```python
from build123d import *

# Parameters (mm, degrees)
F0_W     = 51
F0_H     = 30
F1_DEPTH = 3.175
F2_W     = 115.3
F2_H     = 72.9
F4_DEPTH = 25.4
F3_W     = 115.3
F3_H     = 72.9
F5_DEPTH = 25.4
F6_R     = 0.5
F7_DEPTH = 25


with BuildPart() as f1:
    # F0 (on Top) → F1 (new body)
    with BuildSketch(Plane.XY):
        with BuildLine():
            Line((61, 42.8), (-61, 42.8))
            ThreePointArc((-61, 42.8), (-63.1213203436, 41.9213203436), (-64, 39.8))
            Line((-64, 39.8), (-64, -39.8))
            ThreePointArc((-64, -39.8), (-63.1213203436, -41.9213203436), (-61, -42.8))
            Line((-61, -42.8), (61, -42.8))
            ThreePointArc((61, -42.8), (63.1213203436, -41.9213203436), (64, -39.8))
            Line((64, -39.8), (64, 39.8))
            ThreePointArc((64, 39.8), (63.1213203436, 41.9213203436), (61, 42.8))
        make_face()
        Rectangle(F0_W, F0_H, mode=Mode.SUBTRACT)
    extrude(amount=F1_DEPTH)

    # F2 (on Top) → F4 (join)
    with BuildSketch(Plane.XY):
        with BuildLine():
            Line((-63.9396576047, -36.1556038049), (-57.5896576047, -36.1556038049))
            Line((-57.5896576047, -36.1556038049), (-57.5896576047, -42.5056038049))
            Line((-57.5896576047, -42.5056038049), (61.0603423953, -42.5056038049))
            ThreePointArc((61.0603423953, -42.5056038049), (63.1816627389, -41.6269241484), (64.0603423953, -39.5056038049))
            Line((64.0603423953, -39.5056038049), (64.0603423953, -36.1556038049))
            Line((64.0603423953, -36.1556038049), (64.0603423953, 36.7443961951))
            Line((64.0603423953, 36.7443961951), (64.0603423953, 40.0943961951))
            ThreePointArc((64.0603423953, 40.0943961951), (63.1816627389, 42.2157165387), (61.0603423953, 43.0943961951))
            Line((61.0603423953, 43.0943961951), (-57.5896576047, 43.0943961951))
            Line((-57.5896576047, 43.0943961951), (-60.9396576047, 43.0943961951))
            ThreePointArc((-60.9396576047, 43.0943961951), (-63.0609779483, 42.2157165387), (-63.9396576047, 40.0943961951))
            Line((-63.9396576047, 40.0943961951), (-63.9396576047, -36.1556038049))
        make_face()
        with Locations((0.0603423953, 0.2943961951)):
            Rectangle(F2_W, F2_H, mode=Mode.SUBTRACT)
        with Locations((0.0603423953, 0.2943961951)):
            Rectangle(F2_W, F2_H)
    extrude(amount=-F4_DEPTH)

    # F3 (on Top) → F5 (cut)
    with BuildSketch(Plane.XY):
        Rectangle(F3_W, F3_H)
    extrude(amount=-F5_DEPTH, mode=Mode.SUBTRACT)

    # F6 (on face) → F7 (cut)
    with BuildSketch(Plane(origin=(0, 43.0943961951, 0), x_dir=(-1, 0, 0), z_dir=(0, 1, 0))):
        with Locations((0, -14.8937767372)):
            Circle(F6_R)
    extrude(amount=-F7_DEPTH, mode=Mode.SUBTRACT)


solid = f1.part
```
Geometry check sheet. Reference: the model listing, model coordinates, mm. A direction names the side the tool comes from. Coordinates: 2 decimals unless noted, no trailing zeros. Write each loop counter-clockwise with the first axis right and the second up, starting at its lowest first coordinate (ties: lowest second). Pieces come first, ordered by that corner, then holes. Notation, with made-up numbers: M 51,-18.75 L 109,-18.75 A17 cw 109,12.25 Z; hole C -11.75,-30.5 d2. An arc over 180 degrees is marked long. Use one line per item in the form item = value. Start each with the question number.
1) Section check D-D on z = -3. Enter the section's corners in (x, y).
2) Thickness scan on probe 1 along X at (y, z) = (-15.5, -4.5); probe 2 along Y at (x, z) = (-28, -21.75); probe 3 along Z at (x, y) = (0, 41.75) (3 decimals). Record the ranges inside material, lowest first. Write a range as from..to.
3) Section check C-C on y = 35. Enter the section's corners in (x, z) (3 decimals), and give its area (3 significant figures).
4) Go/stop test with flat-tipped pins: pin 1 Ø7.5 at (x, z) = (-27, -9.5) entering from -Y; pin 2 Ø1 at (y, z) = (-9.5, 1) entering from +X; pin 3 Ø6 at (x, y) = (40.5, -33) entering from -Z. Record where each tip stops, or that it passes through.
5) Section check B-B on x = -44.5. Enter the section's corners in (y, z) (3 decimals), and give its area (3 significant figures).
6) Section check A-A on x = -13.5. Enter the section's corners in (y, z) (3 decimals).
7) Set-up check for faces 5 (the flat face through (1, -42.506, -13)), 6 (the cylindrical face through (63.14, 41.9, 1.57)), 7 (the flat face through (25.5, 0, 2)), 8 (the flat face through (-57.59, -39, -13)), 9 (the cylindrical face through (-63.1, 41.94, 1.57)): record each of +Z, -Z, +X, -X, +Y, -Y from which the full face is reachable in a straight line by a thin tool's end or side.
8) Release check for a two-part mould opening along X. For faces 1 (the flat face through (-57.65, 0, -13)), 2 (the cylindrical face through (-63.14, -41.9, 1.57)), 3 (the flat face through (0, -15, 2)), 4 (the flat face through (-1, -36.45, -13)) record: pulls with the +X half, pulls with the -X half, needs draft (parallel to the pull), parting line crosses it, or undercut.
Responses:
q1.outline = M -63.94,-36.16 L -57.65,-36.16 L -57.65,36.45 L 57.65,36.45 L 57.65,-36.45 L -57.59,-36.45 L -57.59,-42.51 L 61.06,-42.51 A3 ccw 64.06,-39.51 L 64.06,40.09 A3 ccw 61.06,43.09 L -60.94,43.09 A3 ccw -63.94,40.09 Z
q2.probe_1 = -63.94..-57.65, 57.65..64.06
q2.probe_2 = -42.51..-36.45, 36.45..43.09
q2.probe_3 = -25.4..-15.394, -14.394..3.175
q3.outline = M -64,0 L -63.94,0 L -63.94,-25.4 L -57.65,-25.4 L -57.65,0 L 57.65,0 L 57.65,-25.4 L 64.06,-25.4 L 64.06,0 L 64,0 L 64,3.175 L -64,3.175 Z
q3.area = 729 mm2
q4.pin_1 = -42.51
q4.pin_2 = 64
q4.pin_3 = 0
q5.outline = M -42.8,0 L -42.506,0 L -42.506,-25.4 L -36.45,-25.4 L -36.45,0 L 36.45,0 L 36.45,-25.4 L 43.094,-25.4 L 43.094,0 L 42.8,0 L 42.8,3.175 L -42.8,3.175 Z
q5.area = 594 mm2
q6.outline = M -42.8,0 L -42.506,0 L -42.506,-25.4 L -36.45,-25.4 L -36.45,0 L -15,0 L -15,3.175 L -42.8,3.175 Z; M 15,0 L 36.45,0 L 36.45,-25.4 L 43.094,-25.4 L 43.094,0 L 42.8,0 L 42.8,3.175 L 15,3.175 Z
q7.face_5 = -Z, +X, -X, -Y
q7.face_6 = +Z, +X, +Y
q7.face_7 = +Z, -Z
q7.face_8 = -Z, -X, -Y
q7.face_9 = +Z, -X, +Y
q8.face_1 = undercut
q8.face_2 = pulls with the -X half
q8.face_3 = undercut
q8.face_4 = needs draft
